Design review of the part built by this model. Coordinates are the model's own, in mm. Round coordinates to 2 decimals unless told otherwise and drop trailing zeros. Loops run counter-clockwise (first coordinate to the right, second up) from the corner with the lowest first, then second, coordinate; pieces in that order, holes last. Notation, with made-up numbers: (-19.5, 88) -> (32.5, 88) arc R28 cw to (32.5, 114) -> close; hole circle Ø6 at (-7, -7.5). An arc over 180 degrees is marked (long way). Answer as CSV lines item,"result". Start each with the question number.
(1) Take a section at A-A, the plane x = 171. Write out the cut boundary in (y, z), and give its area (3 significant figures).
(2) Take a section at D-D, the plane x = 157. Write out the cut boundary in (y, z).
(3) Take a section at C-C, the plane y = 2.25. Write out the cut boundary in (x, z), and give its area (3 significant figures).
(4) To check wall thickness, follow line 1 (Y direction, x = 173, z = 1049.5); line 2 (Z direction, x = 173, y = 1.25); line 3 (Y direction, x = 124, z = 1058.5). State the ranges of each line that lie inside material, in increasing order. Write a range as from..to.
(5) For P1, Ø10, axis at x = 209, z = 1055, coming from the +Y side, flat-tipped, find the tip position at first contact; note if it passes through.
(6) Take a section at B-B, the plane z = 1053. Write out the cut boundary in (x, y).
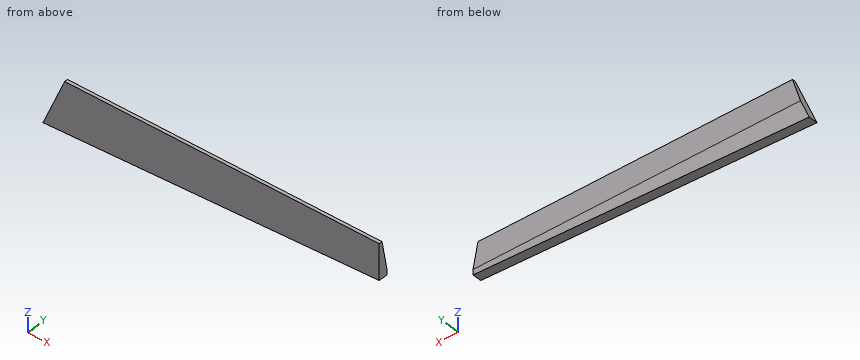
from build123d import *

# Parameters (mm, degrees)
BOSS_EXTRUDE1_DEPTH = 3.81
CHAMFER1_SIZE       = 12.54
CHAMFER1_SIZE2      = 2.437529077


with BuildPart() as part:
    # Sketch2 → Boss-Extrude1 (new body)
    with BuildSketch(Plane(origin=(0, 0, 0), x_dir=(1, 0, 0), z_dir=(0, 1, 0))):
        Polygon((98.033263401, -1041.106556332), (107.044429893, -1061.974520841), (237.469208074, -1061.974520841), (237.469208074, -1047.272091301), align=None)
    extrude(amount=BOSS_EXTRUDE1_DEPTH)

    # Chamfer1
    chamfer1_edges = [part.edges().sort_by_distance(p)[0] for p in [
        (172.256818983, 3.81, 1061.974520841),
    ]]
    chamfer1_side = [part.faces().sort_by_distance(p)[0] for p in [
        (166.193416202, 3.81, 1052.913037199),
    ]]
    chamfer(chamfer1_edges, length=CHAMFER1_SIZE, length2=CHAMFER1_SIZE2, reference=chamfer1_side[0])


solid = part.part
The answers:
1,outline,"(0, 1044.33) -> (3.81, 1044.33) -> (3.81, 1049.43) -> (1.37, 1061.97) -> (0, 1061.97) -> close"
1,area,"51.9 mm²"
2,outline,"(0, 1043.71) -> (3.81, 1043.71) -> (3.81, 1049.43) -> (1.37, 1061.97) -> (0, 1061.97) -> close"
3,outline,"(98.03, 1041.11) -> (237.47, 1047.27) -> (237.47, 1057.46) -> (105.09, 1057.46) -> close"
3,area,"1,790 mm²"
4,line 1,"0..3.8"
4,line 2,"1044.42..1061.97"
4,line 3,"0..2.05"
5,P1,"y = 3.7"
6,outline,"(103.17, 0) -> (237.47, 0) -> (237.47, 3.12) -> (103.17, 3.12) -> close"
